Check sheet for the modelled part. Datum: model origin and axes. Units: mm. A direction names the side the tool comes from. Coordinates: 2 decimals unless noted, no trailing zeros. Write each loop counter-clockwise with the first axis right and the second up, starting at its lowest first coordinate (ties: lowest second). Pieces come first, ordered by that corner, then holes. Notation, with made-up numbers: (81, 65.25) -> (106, 65.25) arc R22 cw to (106, 80.25) -> close; hole circle Ø6 at (59.5, -6.75). An arc over 180 degrees is marked (long way). Put each result on its own line as item: value.
Autodesk Inventor part; units mm, degrees
ref_plane "YZ Plane" through (0, 0, 0) normal (1, 0, 0) x (0, 1, 0)
ref_plane "XZ Plane" through (0, 0, 0) normal (0, 1, 0) x (-1, 0, 0)
ref_plane "XY Plane" through (0, 0, 0) normal (0, 0, 1) x (1, 0, 0)
sketch "Эскиз1" plane through (0, 0, 0) normal (0, 1, 0) x (-1, 0, 0)
  line L0 (-145, 145) -> (145, 145)
  line L1 (145, 145) -> (145, -145)
  line L2 (145, -145) -> (-145, -145)
  line L3 (-145, -145) -> (-145, 145)
  line L4 (145, 0) -> (-145, 0) construction
  line L5 (0, 145) -> (0, -145) construction
  line L6 (145, 145) -> (-145, 145)
  line L7 (-145, 145) -> (-145, 165)
  line L8 (-145, 165) -> (145, 165)
  line L9 (145, 165) -> (145, 145)
  line L10 (145, -145) -> (-145, -145)
  line L11 (-145, -145) -> (-145, -165)
  line L12 (-145, -165) -> (145, -165)
  line L13 (145, -165) -> (145, -145)
  point P0 (0, 0)
  point P1 (0, 0)
  dimension "d0" = 290
  dimension "d1" = 290
  dimension "d2" = 290
  dimension "d3" = 20
  dimension "d4" = 290
  dimension "d5" = 20
extrude "Выдавливание1" add sketch "Эскиз1" along normal blind 5 contours L0 L1 L2 L3
extrude "Выдавливание2" add sketch "Эскиз1" along normal blind 155 contours L7 L8 L9 L0 | L2 L13 L12 L11
sketch "Эскиз2" plane through (145, 5, 145) normal (0, 0, -1) x (-1, 0, 0)
  line L0 (0, -5) -> (0, 150)
  line L1 (0, -5) -> (290, -5)
  line L2 (290, -5) -> (290, 0)
  line L3 (290, 0) -> (0, 0)
  line L4 (0, 0) -> (0, -5)
  line L5 (145, 0) -> (145, 150) construction
  line L6 (290, 150) -> (0, 150)
  line L7 (145, 0) -> (145, 70) construction
  line L8 (145, 0) -> (145, 20) construction
  line L9 (145, 20) -> (0, 20)
  line L10 (0, 20) -> (0, 120)
  line L11 (0, 120) -> (145, 120)
  line L12 (145, 120) -> (145, 20)
  line L13 (145, 20) -> (290, 20)
  line L14 (290, 20) -> (290, 120)
  line L15 (290, 120) -> (145, 120)
  line L16 (145, 120) -> (145, 20)
  point P0 (145, -5)
  dimension "d10" = 290
  dimension "d11" = 5
  dimension "d12" = 70
  dimension "d13" = 20
  dimension "d14" = 145
  dimension "d15" = 100
  dimension "d16" = 145
  dimension "d17" = 100
properties part number "maze_test_course"
Q1. Material ranges on line 1 along Z through (x, y) = (128, 114); line 2 along Y through (x, z) = (3, 115.5), recorded low to high.
Recorded:
line 1: z = -165 to -145, 145 to 165
line 2: y = 0 to 5
Q2. Cross-section at A-A (y = 108.5). Record the cut outline in (x, z), plus the area to 3 significant figures.
Recorded:
outline: (-145, -165) -> (145, -165) -> (145, -145) -> (-145, -145) -> close; (-145, 145) -> (145, 145) -> (145, 165) -> (-145, 165) -> close
area: 11,600 mm2
Q3. Tool access check on faces 1 (the flat face through (-145, 3, 1)), 2 (the flat face through (2, 79, 145)). Record the directions out of +Z, -Z, +X, -X, +Y, -Y that give a thin tool (end or side, any length) a straight path to the whole face; none if there is none.
Recorded:
face 1: +Z, -Z, -X, +Y, -Y
face 2: +X, -X, +Y
Q4. Cross-section at B-B (x = -0.5). Record the cut outline in (y, z).
Recorded:
outline: (0, -165) -> (155, -165) -> (155, -145) -> (5, -145) -> (5, 145) -> (155, 145) -> (155, 165) -> (0, 165) -> close
Q5. Cross-section at C-C (z = 101). Record the cut outline in (x, y).
Recorded:
outline: (-145, 0) -> (145, 0) -> (145, 5) -> (-145, 5) -> close
Q6. Mould release check, pull along Z, two halves, no side actions. Record for faces 3 (the flat face through (2, 5, 2)), 4 (the flat face through (2, 76, 165)), 5 (the flat face through (2, 0, 2)): released by +Z, released by -Z, zero draft, split by the parting line, or undercut.
Recorded:
face 3: undercut
face 4: released by +Z
face 5: zero draft
Q7. Depth check by flat-ended pin: P1, Ø3, axis at x = -52, z = -108.5, coming from the +Y side; P2, Ø1, axis at x = -59.5, z = 108, coming from the -Y side. Enter the tip coordinate at first touch or a pass-through.
Recorded:
P1: stops at y = 5
P2: stops at y = 0
